from build123d import *

# Parameters (mm, degrees)
CROQUIS1_R              = 1.75
SALIENTE_EXTRUIR1_DEPTH = 10
CROQUIS3_W              = 40
CROQUIS3_H              = 20
SALIENTE_EXTRUIR2_DEPTH = 10
CROQUIS4_R              = 2.25
CORTAR_EXTRUIR2_DEPTH   = 10
CORTAR_EXTRUIR3_DEPTH   = 1
CROQUIS6_R              = 3.6
CORTAR_EXTRUIR4_DEPTH   = 4.3


with BuildPart() as part:
    # Croquis1 → Saliente-Extruir1 (new body)
    with BuildSketch(Plane.XY):
        with BuildLine():
            Line((0, 6), (31, 6))
            Line((31, 6), (37, 6))
            Line((37, 6), (37, 0))
            Line((37, 0), (37, -31))
            ThreePointArc((37, -31), (31, -37), (25, -31))
            Line((25, -31), (25, -21.980740698))
            ThreePointArc((25, -21.980740698), (23.631727984, -7.368272016), (9.019259302, -6))
            Line((9.019259302, -6), (0, -6))
            ThreePointArc((0, -6), (-6, 0), (0, 6))
        make_face()
        Circle(CROQUIS1_R, mode=Mode.SUBTRACT)
        with Locations((31, 0)):
            Circle(CROQUIS1_R, mode=Mode.SUBTRACT)
        with Locations((31, -31)):
            Circle(CROQUIS1_R, mode=Mode.SUBTRACT)
    extrude(amount=SALIENTE_EXTRUIR1_DEPTH)

    # Croquis3 → Saliente-Extruir2 (add)
    with BuildSketch(Plane(origin=(37, 0, 0), x_dir=(0, 0, -1), z_dir=(1, 0, 0))):
        with Locations((-5, -4)):
            Rectangle(CROQUIS3_W, CROQUIS3_H)
    extrude(amount=SALIENTE_EXTRUIR2_DEPTH)

    # Croquis4 → Cortar-Extruir2 (cut)
    with BuildSketch(Plane(origin=(47, 0, 0), x_dir=(0, 0, -1), z_dir=(1, 0, 0))):
        with Locations((-17.5, -4)):
            Circle(CROQUIS4_R)
        with Locations((7.5, -4)):
            Circle(CROQUIS4_R)
    extrude(amount=-CORTAR_EXTRUIR2_DEPTH, mode=Mode.SUBTRACT)

    # Croquis5 → Cortar-Extruir3 (cut)
    # profile 1 of 2: a face of its own
    with BuildSketch(Plane(origin=(0, 6, 0), x_dir=(1, 0, 0), z_dir=(0, 1, 0))):
        with BuildLine():
            Line((38.719450651, -5.423076923), (39.045171805, -5.008413462))
            Line((39.045171805, -5.008413462), (41.469450651, -6.59375))
            add(Edge.make_bspline(
                [(41.469450651, -6.59375), (41.45262689, -6.488200954), (41.419810241, -6.282315605), (41.414396621, -6.073916922), (41.411758343, -5.972355769)],
                knots=[0, 0, 0, 0, 1.025318673, 2, 2, 2, 2], degree=3))
            add(Edge.make_bspline(
                [(41.411758343, -5.972355769), (41.413397392, -5.911374347), (41.41662381, -5.791334232), (41.441453269, -5.615094001), (41.48058203, -5.445741533), (41.537620193, -5.283978793), (41.610481332, -5.12922502), (41.69780526, -4.98059268), (41.804100137, -4.84087365), (41.922842279, -4.708276629), (42.054348853, -4.587868709), (42.193923862, -4.481348491), (42.341556266, -4.391383269), (42.497212867, -4.319707477), (42.659675206, -4.262425826), (42.829576898, -4.221648263), (43.0072047, -4.197270821), (43.128028028, -4.193979555), (43.189402574, -4.192307692)],
                knots=[0, 0, 0, 0, 1.043709831, 2.054511743, 3.041122595, 4.01515914, 4.98481438, 5.965901842, 6.960491961, 7.985277438, 9.0096037, 10.00832444, 10.987059228, 11.962929573, 12.936966118, 13.931840027, 14.949438142, 16, 16, 16, 16], degree=3))
            add(Edge.make_bspline(
                [(43.189402574, -4.192307692), (43.273370923, -4.194741372), (43.438600762, -4.199530277), (43.679201656, -4.247450052), (43.908280527, -4.321356873), (44.121873475, -4.428685672), (44.321459866, -4.559473328), (44.497723912, -4.720926587), (44.654923346, -4.905035031), (44.786320549, -5.113320498), (44.893643904, -5.337445219), (44.970726157, -5.572907398), (45.018183801, -5.817410653), (45.024133369, -5.983361467), (45.027142959, -6.067307692)],
                knots=[0, 0, 0, 0, 1.031403119, 2.029557249, 3.004870281, 3.983165322, 4.960181699, 5.929903783, 6.912123683, 7.928973898, 8.949315281, 9.960468141, 10.968302741, 12, 12, 12, 12], degree=3))
            add(Edge.make_bspline(
                [(45.027142959, -6.067307692), (45.024530622, -6.148048292), (45.019356041, -6.307981282), (44.973019832, -6.5431878), (44.898450918, -6.769592811), (44.79356478, -6.984290092), (44.66331814, -7.183504791), (44.507611369, -7.363156395), (44.32622815, -7.5184301), (44.123136349, -7.648813278), (43.905204402, -7.75266345), (43.677571617, -7.829814545), (43.441193643, -7.875117968), (43.280937295, -7.881434097), (43.200219882, -7.884615385)],
                knots=[0, 0, 0, 0, 1.012172929, 2.004937354, 2.995255351, 3.995689452, 4.993936421, 5.973737378, 6.968231049, 7.979117505, 8.993136101, 9.989812463, 10.987515067, 12, 12, 12, 12], degree=3))
            add(Edge.make_bspline(
                [(43.200219882, -7.884615385), (43.138429168, -7.88259005), (43.012264336, -7.878454705), (42.821183145, -7.849580321), (42.625667005, -7.80318353), (42.459802673, -7.751223108), (42.323925778, -7.696322062), (42.214376937, -7.650631994), (42.101643669, -7.593762287), (41.981860293, -7.533122205), (41.858113837, -7.463253287), (41.728336117, -7.387283602), (41.594591099, -7.303112772), (41.503829621, -7.244106778), (41.45743142, -7.213942308)],
                knots=[0, 0, 0, 0, 1.173818275, 2.396712641, 3.66331629, 4.989737886, 5.693666774, 6.447286557, 7.243889047, 8.091586357, 8.998013824, 9.943181721, 10.948533338, 12, 12, 12, 12], degree=3))
            Line((41.45743142, -7.213942308), (38.719450651, -5.423076923))
        make_face()
        with BuildLine():
            add(Edge.make_bspline(
                [(42.027142959, -6.085336538), (42.028463871, -6.131047697), (42.031043996, -6.220334868), (42.046353115, -6.351256722), (42.074217455, -6.47556773), (42.112853793, -6.593303975), (42.160487874, -6.705191769), (42.221606583, -6.809013804), (42.29279593, -6.906906504), (42.373927128, -6.997305799), (42.462694986, -7.079287189), (42.557788622, -7.149882157), (42.656897901, -7.210778026), (42.760855723, -7.260289629), (42.869621095, -7.298844068), (42.982694109, -7.326732492), (43.100832915, -7.34225321), (43.180945778, -7.344835321), (43.221854497, -7.346153846)],
                knots=[0, 0, 0, 0, 1.129656352, 2.206547016, 3.251334079, 4.271920891, 5.265058649, 6.249872215, 7.241923875, 8.251504132, 9.246416584, 10.222533834, 11.173322129, 12.116503788, 13.062124155, 14.020151864, 14.989013135, 16, 16, 16, 16], degree=3))
            add(Edge.make_bspline(
                [(43.221854497, -7.346153846), (43.262390236, -7.345042059), (43.342270883, -7.342851147), (43.459527516, -7.324197734), (43.572108371, -7.294382199), (43.679590351, -7.251311648), (43.784036826, -7.19897235), (43.882187361, -7.131790832), (43.97722126, -7.054685968), (44.064722932, -6.964658995), (44.145955918, -6.8673042), (44.217253031, -6.763510182), (44.277542135, -6.654839733), (44.327498317, -6.541605832), (44.364273193, -6.422408765), (44.39242636, -6.29918399), (44.407818081, -6.170256123), (44.410427684, -6.082969666), (44.411758343, -6.038461538)],
                knots=[0, 0, 0, 0, 0.989367052, 1.949669134, 2.891858276, 3.827522767, 4.772653562, 5.738670152, 6.725809442, 7.756636004, 8.798867547, 9.819240912, 10.826537776, 11.829883227, 12.835515726, 13.868058748, 14.912904531, 16, 16, 16, 16], degree=3))
            add(Edge.make_bspline(
                [(44.411758343, -6.038461538), (44.41042758, -5.993953484), (44.407817774, -5.90666717), (44.392427526, -5.777738265), (44.364268919, -5.654517323), (44.327513802, -5.535306334), (44.277484342, -5.422124068), (44.217630322, -5.313548608), (44.145518764, -5.210736256), (44.064862408, -5.113318104), (43.976721258, -5.02366527), (43.883043664, -4.944746981), (43.783251472, -4.879664359), (43.680001032, -4.825249844), (43.572044173, -4.782656193), (43.459545037, -4.752693871), (43.342266312, -4.73408014), (43.262388698, -4.731883781), (43.221854497, -4.730769231)],
                knots=[0, 0, 0, 0, 1.087281468, 2.132306021, 3.165025708, 4.170830268, 5.174347389, 6.181816599, 7.194310624, 8.23672049, 9.267723423, 10.261267456, 11.222032883, 12.171822355, 13.107646935, 14.049997283, 15.01046367, 16, 16, 16, 16], degree=3))
            add(Edge.make_bspline(
                [(43.221854497, -4.730769231), (43.180892409, -4.73171259), (43.100497153, -4.733564098), (42.982746954, -4.754505725), (42.869046586, -4.783549789), (42.760110728, -4.827406434), (42.656368933, -4.884383287), (42.557298409, -4.953783726), (42.462134709, -5.034066908), (42.373753422, -5.126810316), (42.292883888, -5.227746884), (42.22170449, -5.335154265), (42.160945465, -5.447073949), (42.113001784, -5.565082488), (42.074377809, -5.687592088), (42.046452462, -5.815448694), (42.031083903, -5.948743241), (42.028473339, -6.039225506), (42.027142959, -6.085336538)],
                knots=[0, 0, 0, 0, 0.978259475, 1.920005202, 2.851759169, 3.7803069, 4.719124913, 5.675758531, 6.668034766, 7.691045932, 8.733780038, 9.756656648, 10.768121246, 11.773215211, 12.79725739, 13.836288844, 14.897342417, 16, 16, 16, 16], degree=3))
        make_face(mode=Mode.SUBTRACT)
    # profile 2 of 2: a face of its own
    with BuildSketch(Plane(origin=(0, 6, 0), x_dir=(1, 0, 0), z_dir=(0, 1, 0))):
        with BuildLine():
            add(Edge.make_bspline(
                [(43.950219882, -2.615384615), (43.95220531, -2.581972823), (43.956097511, -2.51647291), (43.98280038, -2.421777262), (44.030215227, -2.336072131), (44.093408561, -2.25973114), (44.170029698, -2.196805752), (44.255051256, -2.147701148), (44.3505397, -2.121230888), (44.416419143, -2.117367039), (44.450219882, -2.115384615)],
                knots=[0, 0, 0, 0, 1.020151414, 1.999887582, 2.974338812, 3.990962822, 5.007586832, 5.987933904, 6.967670073, 8, 8, 8, 8], degree=3))
            add(Edge.make_bspline(
                [(44.450219882, -2.115384615), (44.48321411, -2.117427904), (44.548278244, -2.121457239), (44.642964488, -2.147713091), (44.728083557, -2.196746141), (44.804525099, -2.260131503), (44.869244769, -2.335615588), (44.916031001, -2.422045399), (44.944737682, -2.516233448), (44.948370129, -2.581929945), (44.950219882, -2.615384615)],
                knots=[0, 0, 0, 0, 1.009624703, 1.990965087, 2.972917375, 3.991206001, 5.017354006, 5.993400798, 6.978178195, 8, 8, 8, 8], degree=3))
            add(Edge.make_bspline(
                [(44.950219882, -2.615384615), (44.948437276, -2.648863379), (44.944957162, -2.714222696), (44.915444253, -2.80805959), (44.869691223, -2.895016193), (44.804407281, -2.970480663), (44.728478959, -3.034379676), (44.642378281, -3.081237346), (44.548549602, -3.109769691), (44.483267561, -3.113497493), (44.450219882, -3.115384615)],
                knots=[0, 0, 0, 0, 1.022258411, 1.995716197, 2.98297171, 4.009558169, 5.028281891, 6.00474573, 6.989943903, 8, 8, 8, 8], degree=3))
            add(Edge.make_bspline(
                [(44.450219882, -3.115384615), (44.416363802, -3.113563874), (44.350263962, -3.110009099), (44.255636921, -3.081250825), (44.169633882, -3.034320176), (44.093525459, -2.970882356), (44.029775797, -2.894554991), (43.983379009, -2.808332925), (43.95588116, -2.713979428), (43.952139702, -2.648819533), (43.950219882, -2.615384615)],
                knots=[0, 0, 0, 0, 1.032775665, 2.016367738, 2.991239715, 4.008302682, 5.025365648, 6.011011707, 6.979408107, 8, 8, 8, 8], degree=3))
        make_face()
    extrude(amount=-CORTAR_EXTRUIR3_DEPTH, mode=Mode.SUBTRACT)

    # Croquis6 → Cortar-Extruir4 (cut)
    with BuildSketch(Plane.ZY.offset(-37)):
        with Locations((-7.5, -4)):
            Circle(CROQUIS6_R)
    extrude(amount=-CORTAR_EXTRUIR4_DEPTH, mode=Mode.SUBTRACT)


solid = part.part
Geometry: final body of the model. Coordinates: model frame, mm. A direction names the side the tool comes from. Give positions to 0.01 mm unless a question says otherwise; leave off trailing zeros. Write each loop counter-clockwise with the first axis right and the second up, starting at its lowest first coordinate (ties: lowest second). Pieces come first, ordered by that corner, then holes.
(1) Cut plane A-A, the plane z = 17.5. Return loops of the section in (x, y).
(2) Access query for faces 1 (the cylindrical face through (39.12, -5.379, -4.175)), 2 (the flat face through (25, -6, 0)), 3 (the flat face through (37, -1.6, 17.6)). Directions: +Z, -Z, +X, -X, +Y, -Y. A direction counts if a zero-diameter tool reaches every point of the face in a straight line with its end or side. Return the directions, or none.
(3) Cut plane B-B, the plane x = -1. Return loops of the section in (y, z).
(4) First-contact query: P1, Ø8, axis at y = -20.5, z = -0.5, coming from the -X side; P2, Ø10, axis at y = -12.5, z = 5.5, coming from the -X side; P3, Ø2, axis at y = -2, z = -2, coming from the -X side. Flat tips, straight axial feed; report the tip coordinate or a pass-through.
(5) Cut plane C-C, the plane z = 9. Return loops of the section in (x, y).
(6) Cut plane D-D, the plane y = -11. Return loops of the section in (x, z).
(7) Ray query, line 1 (Y direction, x = 31, z = 6); line 2 (Y direction, x = 40.1, z = -7.5); line 3 (Y direction, x = 44.75, z = 17.5). Return the intervals inside material, ascending.
(8) Mould query, pull axis Z, two halves, no side actions, for faces 4 (the cylindrical face through (44.19, -5.369, -5.714)), 5 (the flat face through (42, -4, -15)), 6 (the cylindrical face through (29.25, -30.92, 4.93)). Classes: released by +Z, released by -Z, zero draft, split by the parting line, or undercut.
Values follow:
1. outline: (37, -14) - (47, -14) - (47, -6.25) - (37, -6.25) - close; (37, -1.75) - (47, -1.75) - (47, 6) - (37, 6) - close
2. face 1: -X
2. face 2: -Z, -X, +Y, -Y
2. face 3: +Z, -X, +Y, -Y
3. outline: (-5.92, 0) - (-1.44, 0) - (-1.44, 10) - (-5.92, 10) - close; (1.44, 0) - (5.92, 0) - (5.92, 10) - (1.44, 10) - close
4. P1: stops at x = 25
4. P2: stops at x = 23.76
4. P3: stops at x = 37
5. outline: (0, -6) - (9.02, -6) arc R11.5 cw to (25, -21.98) - (25, -31) arc R6 ccw to (37, -31) - (37, -14) - (47, -14) - (47, 6) - (0, 6) arc R6 ccw to start; hole circle Ø3.5 at (0, 0); hole circle Ø3.5 at (31, -31); hole circle Ø3.5 at (31, 0)
6. outline: (26.08, 0) - (37, 0) - (37, -15) - (47, -15) - (47, 25) - (37, 25) - (37, 10) - (26.08, 10) - close
7. line 1: y = -37 to -32.75, -29.25 to -1.75, 1.75 to 6
7. line 2: y = -14 to -7.6, -0.4 to 6
7. line 3: y = -14 to -6.25, -1.75 to 6
8. face 4: undercut
8. face 5: released by -Z
8. face 6: zero draft
